Work out the finished part from the listing and answer in its coordinate system (mm). Round coordinates to 2 decimals unless told otherwise and drop trailing zeros. Write each loop counter-clockwise with the first axis right and the second up, starting at its lowest first coordinate (ties: lowest second). Pieces come first, ordered by that corner, then holes. Notation, with made-up numbers: (-10.75, 65.25) -> (40.25, 65.25) arc R10 cw to (40.25, 71.25) -> close; hole circle Ø3 at (-2, 75.25). An arc over 180 degrees is marked (long way). Answer as a JSON object with one key per item and string values. Group by question number.
from build123d import *

# Parameters (mm, degrees)
SKETCH1_R           = 187.5
BOSS_EXTRUDE1_DEPTH = 4
SKETCH2_R           = 37
CUT_EXTRUDE1_DEPTH  = 266.195211118
SKETCH3_R           = 1.755
CUT_EXTRUDE2_DEPTH  = 266.195211118
CIRPATTERN1_COUNT   = 20
SKETCH4_R           = 1.755
CUT_EXTRUDE3_DEPTH  = 266.195211118
CIRPATTERN2_COUNT   = 20


with BuildPart() as part:
    # Sketch1 → Boss-Extrude1 (new body)
    with BuildSketch(Plane.XY):
        Circle(SKETCH1_R)
    extrude(amount=BOSS_EXTRUDE1_DEPTH)

    # Sketch2 → Cut-Extrude1 (cut, through all)
    with BuildSketch(Plane.XY.offset(4)):
        Circle(SKETCH2_R)
    extrude(amount=-CUT_EXTRUDE1_DEPTH, mode=Mode.SUBTRACT)

    # Sketch3 → Cut-Extrude2 (cut, through all)
    with BuildSketch(Plane.XY.offset(4)):
        with Locations((0, 175)):
            Circle(SKETCH3_R)
    cut_extrude2 = extrude(amount=-CUT_EXTRUDE2_DEPTH, mode=Mode.SUBTRACT)

    # CirPattern1: Cut-Extrude2 ×20 about axis
    cirpattern1_axis = Axis((0, 0, 0), (0, 0, 1))
    for i in range(1, CIRPATTERN1_COUNT):
        add(cut_extrude2.rotate(cirpattern1_axis, i * 360 / CIRPATTERN1_COUNT), mode=Mode.SUBTRACT)

    # Sketch4 → Cut-Extrude3 (cut, through all)
    with BuildSketch(Plane(origin=(0, 0, 0), x_dir=(-1, 0, 0), z_dir=(0, 0, -1))):
        with Locations((-12.959885154, -81.825494522)):
            Circle(SKETCH4_R)
        with Locations((-20.781608406, -131.209911552)):
            Circle(SKETCH4_R)
    cut_extrude3 = extrude(amount=-CUT_EXTRUDE3_DEPTH, mode=Mode.SUBTRACT)

    # CirPattern2: Cut-Extrude3 ×20 about axis
    cirpattern2_axis = Axis((0, 0, 0), (0, 0, 1))
    for i in range(1, CIRPATTERN2_COUNT):
        add(cut_extrude3.rotate(cirpattern2_axis, i * 360 / CIRPATTERN2_COUNT), mode=Mode.SUBTRACT)


solid = part.part
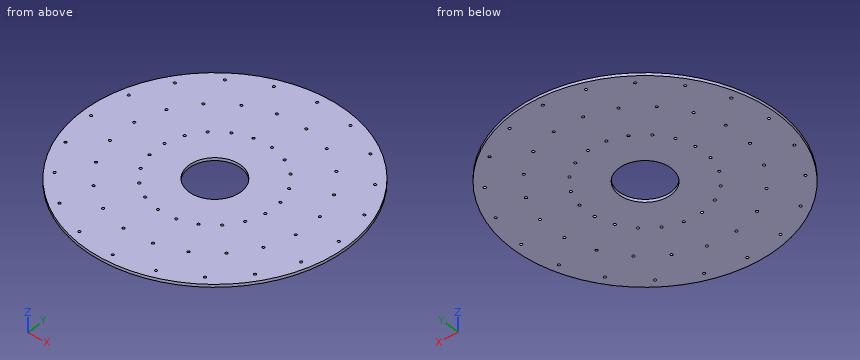
1) A cutting plane is placed at B-B on y = -67. Determine the outline of the cut face in (x, z), plus the area to 3 significant figures.
2) Straight lines are drawn through the part: L1, parallel to Y at x = 0, z = 2.25 (3 decimals); L2, parallel to X at y = -55.5, z = 0.35; L3, parallel to X at y = 131, z = 2.75. For each, find the intervals that lie inside material, in ascending order.
3) A cutting plane is placed at A-A on z = 2.5. State how many separate pieces and enclosed holes the cut face has, plus the area to 3 significant figures.
4) Each of these flat-tipped pins is pushed along its axis until it touches: P1, Ø3, axis at x = 60.31, y = -118.37, coming from the -Z side; P2, Ø6, axis at x = 50.5, y = 124, coming from the -Z side; P3, Ø2, axis at x = 36.5, z = 1, coming from the +Y side; P4, Ø2, axis at x = 90.5, z = 1.5, coming from the -Y side. Where does it stop, or does it pass through?
Established:
{
 "1": {"outline": "(-175.12, 0) -> (175.12, 0) -> (175.12, 4) -> (-175.12, 4) -> close", "area": "1,400 mm²"},
 "2": {"L1": "y = -187.5 to -176.755, -173.245 to -37, 37 to 173.245, 176.755 to 187.5", "L2": "x = -179.1 to -167.46, -165.41 to 165.41, 167.46 to 179.1", "L3": "x = -134.15 to -22.52, -19.04 to 19.04, 22.52 to 134.15"},
 "3": {"separate pieces": "1", "enclosed holes": "61", "area": "106,000 mm²"},
 "4": {"P1": "passes through", "P2": "stops at z = 0", "P3": "stops at y = 184.11", "P4": "stops at y = -164.76"}
}
